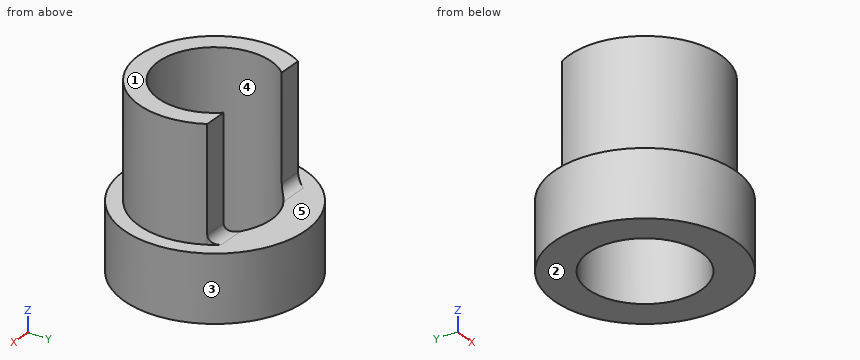
from build123d import *
from build123d.topology import SkipClean

# Parameters (mm, degrees)
BOSS_EXTRUDE1_DEPTH = 3
BOSS_EXTRUDE2_START = 1.75
SKETCH2_R           = 2.4
SKETCH2_R_2         = 1.495
BOSS_EXTRUDE2_DEPTH = 1.75
FILLET1_R           = 0.25


with BuildPart() as part:
    # Sketch1 → Boss-Extrude1 (new body)
    with BuildSketch(Plane.XY):
        with BuildLine():
            Line((-1.737821913, 1), (-1.111316787, 1))
            ThreePointArc((-1.111316787, 1), (0, -1.495), (1.111316787, 1))
            Line((1.111316787, 1), (1.737821913, 1))
            ThreePointArc((1.737821913, 1), (0, -2.005), (-1.737821913, 1))
        make_face()
    extrude(amount=BOSS_EXTRUDE1_DEPTH)

    # Sketch2 → Boss-Extrude2 (add)
    with SkipClean():  # the faces are left unmerged after this step: merging them gives an invalid solid
        with BuildSketch(Plane(origin=(0, 0, 0), x_dir=(-1, 0, 0), z_dir=(0, 0, -1)).offset(BOSS_EXTRUDE2_START)):
            Circle(SKETCH2_R)
            Circle(SKETCH2_R_2, mode=Mode.SUBTRACT)
        extrude(amount=-BOSS_EXTRUDE2_DEPTH)

    # Fillet1
    # the kernel refuses this fillet: 0.25 mm, written as the material it adds along each edge
    with BuildSketch(Plane(origin=(-2.362821913, 1, 0), x_dir=(0, 0, 1), z_dir=(1, 0, 0))) as fillet1_piece_1_section:
        with BuildLine():
            CenterArc((FILLET1_R, -FILLET1_R), FILLET1_R, 90, 90)
            Line((0, -FILLET1_R), (0, 0))
            Line((0, 0), (FILLET1_R, 0))
        make_face()
    fillet1_piece_1 = extrude(amount=1.876505126, mode=Mode.PRIVATE)
    fillet1_piece_1 = fillet1_piece_1 & Plane(origin=(0, 0, 0.055527153), x_dir=(0.8667440960723748, 0.49875311720698257, 0), z_dir=(0, 0, -1)) * Cylinder(2.005, 5, mode=Mode.PRIVATE)
    fillet1_piece_1 = fillet1_piece_1 - Plane(origin=(0, 0, 0.055527153), x_dir=(-0.7433557100464799, 0.6688963210702342, 0), z_dir=(0, 0, -1)) * Cylinder(1.495, 5, mode=Mode.PRIVATE)
    add(fillet1_piece_1)
    with BuildSketch(Plane(origin=(0.486316787, 1, 0), x_dir=(0, 0, 1), z_dir=(1, 0, 0))) as fillet1_piece_2_section:
        with BuildLine():
            CenterArc((FILLET1_R, -FILLET1_R), FILLET1_R, 90, 90)
            Line((0, -FILLET1_R), (0, 0))
            Line((0, 0), (FILLET1_R, 0))
        make_face()
    fillet1_piece_2 = extrude(amount=1.876505126, mode=Mode.PRIVATE)
    fillet1_piece_2 = fillet1_piece_2 & Plane(origin=(0, 0, 0.055527144), x_dir=(0.8667440960723748, 0.49875311720698257, 0), z_dir=(0, 0, -1)) * Cylinder(2.005, 5, mode=Mode.PRIVATE)
    fillet1_piece_2 = fillet1_piece_2 - Plane(origin=(0, 0, 0.055527144), x_dir=(-0.7433557100464799, 0.6688963210702342, 0), z_dir=(0, 0, -1)) * Cylinder(1.495, 5, mode=Mode.PRIVATE)
    add(fillet1_piece_2)


solid = part.part
Source: CAD feature listing. Evaluate the final solid. Frame: model axes, mm. Face numbers are marked on the shaded views. A direction names the side the tool comes from. Round coordinates to 2 decimals unless told otherwise and drop trailing zeros. Loops run counter-clockwise (first coordinate to the right, second up) from the corner with the lowest first, then second, coordinate; pieces in that order, holes last. Notation, with made-up numbers: (85, 26) -> (124, 26) arc R16 ccw to (124, 31) -> close; hole circle Ø8 at (-4, 42.5). An arc over 180 degrees is marked (long way). Answer as a JSON object with one key per item and string values. Group by question number.
Q1. Mould query, pull axis Z, two halves, no side actions, for the marked faces 1, 2 and 3. Classes: pulls with the +Z half, pulls with the -Z half, needs draft (parallel to the pull), parting line crosses it, or undercut.
Q2. Section query B-B (y = -1.1). Output: boundary loops of the cut face in (x, z), plus the area to 3 significant figures.
Q3. Ray query, line 1 (X direction, y = 0, z = 1.35) (3 decimals); line 2 (Y direction, x = 0, z = 0.75) (3 decimals); line 3 (Y direction, x = -1.3, z = -0.5). Return the intervals inside material, ascending. Write a range as from..to.
Q4. Access query for the marked faces 4 and 5. Directions: +Z, -Z, +X, -X, +Y, -Y. A direction counts if a zero-diameter tool reaches every point of the face in a straight line with its end or side. Return the directions, or none.
Q5. Contact query for flat-ended pins moving along their axis: P1, Ø1.8, axis at x = 0, y = 0, coming from the +Z side; P2, Ø0.5, axis at x = 1.5, z = 1, coming from the +Y side; P3, Ø2, axis at y = -1.5, z = -1, coming from the +X side. Output: stop coordinate, or through.
Q6. Section query C-C (z = -1.15). Output: boundary loops of the cut face in (x, y) (3 decimals), plus the area to 3 significant figures.
Q7. Section query D-D (x = 0.9). Output: boundary loops of the cut face in (y, z), plus the area to 3 significant figures.
Q8. Section query A-A (x = 0). Output: boundary loops of the cut face in (y, z) (3 decimals), plus the area to 3 significant figures.
Completed:
{
 "1": {"face 1": "pulls with the +Z half", "face 2": "pulls with the -Z half", "face 3": "needs draft"},
 "2": {"outline": "(-2.13, -1.75) -> (-1.01, -1.75) -> (-1.01, 3) -> (-1.68, 3) -> (-1.68, 0) -> (-2.13, 0) -> close; (1.01, -1.75) -> (2.13, -1.75) -> (2.13, 0) -> (1.68, 0) -> (1.68, 3) -> (1.01, 3) -> close", "area": "7.91 mm²"},
 "3": {"line 1": "-2.005..-1.495, 1.495..2.005", "line 2": "-2.005..-1.495", "line 3": "-2.02..-0.74, 0.74..2.02"},
 "4": {"face 4": "+Z, -Z", "face 5": "+Z"},
 "5": {"P1": "through", "P2": "y = 1", "P3": "x = 2.35"},
 "6": {"outline": "circle Ø4.8 at (0, 0); hole circle Ø2.99 at (0, 0)", "area": "11.1 mm²"},
 "7": {"outline": "(-2.22, -1.75) -> (-1.19, -1.75) -> (-1.19, 3) -> (-1.79, 3) -> (-1.79, 0) -> (-2.22, 0) -> close; (1.19, -1.75) -> (2.22, -1.75) -> (2.22, 0) -> (1.25, 0) arc R0.25 cw to (1.19, 0.01) -> close", "area": "5.40 mm²"},
 "8": {"outline": "(-2.4, -1.75) -> (-1.495, -1.75) -> (-1.495, 3) -> (-2.005, 3) -> (-2.005, 0) -> (-2.4, 0) -> close; (1.495, -1.75) -> (2.4, -1.75) -> (2.4, 0) -> (1.495, 0) -> close", "area": "4.70 mm²"}
}
